from build123d import *

# Parameters (mm, degrees)
SKETCH_1_R      = 2.25
SKETCH_1_R_2    = 4.1
EXTRUDE_1_DEPTH = 1


with BuildPart() as part:
    # 草图1 → 凸台-拉伸1 (new body)
    with BuildSketch(Plane.XY.offset(1)):
        with BuildLine():
            Line((-614.361406616, 5), (-620, 5))
            ThreePointArc((-620, 5), (-622.5, 5.669872981), (-624.330127019, 7.5))
            ThreePointArc((-624.330127019, 7.5), (-625.42820323, 8.598076211), (-626.92820323, 9))
            Line((-626.92820323, 9), (-640, 9))
            ThreePointArc((-640, 9), (-646.363961031, 6.363961031), (-649, 0))
            ThreePointArc((-649, 0), (-600, -49), (-551, 0))
            ThreePointArc((-551, 0), (-553.636038969, 6.363961031), (-560, 9))
            Line((-560, 9), (-573.07179677, 9))
            ThreePointArc((-573.07179677, 9), (-574.57179677, 8.598076211), (-575.669872981, 7.5))
            ThreePointArc((-575.669872981, 7.5), (-577.5, 5.669872981), (-580, 5))
            Line((-580, 5), (-585.638593384, 5))
            ThreePointArc((-585.638593384, 5), (-587.901487472, 3.969596493), (-588.60991889, 1.586206897))
            ThreePointArc((-588.60991889, 1.586206897), (-589.388591149, -4.432606704), (-593.122606779, -9.216911765))
            ThreePointArc((-593.122606779, -9.216911765), (-594.713337054, -9.80559868), (-596.369078113, -9.4375))
            ThreePointArc((-596.369078113, -9.4375), (-600, -8.5), (-603.630921887, -9.4375))
            ThreePointArc((-603.630921887, -9.4375), (-605.286662946, -9.80559868), (-606.877393221, -9.216911765))
            ThreePointArc((-606.877393221, -9.216911765), (-610.611408851, -4.432606704), (-611.39008111, 1.586206897))
            ThreePointArc((-611.39008111, 1.586206897), (-612.098512528, 3.969596493), (-614.361406616, 5))
        make_face()
        with Locations((-640, 0)):
            Circle(SKETCH_1_R, mode=Mode.SUBTRACT)
        with Locations((-600, -30)):
            Circle(SKETCH_1_R_2, mode=Mode.SUBTRACT)
        with Locations((-567.639320225, -23.511410092)):
            Circle(SKETCH_1_R, mode=Mode.SUBTRACT)
        with Locations((-587.639320225, -38.042260652)):
            Circle(SKETCH_1_R, mode=Mode.SUBTRACT)
        with Locations((-612.360679775, -38.042260652)):
            Circle(SKETCH_1_R, mode=Mode.SUBTRACT)
        with Locations((-632.360679775, -23.511410092)):
            Circle(SKETCH_1_R, mode=Mode.SUBTRACT)
        with Locations((-560, 0)):
            Circle(SKETCH_1_R, mode=Mode.SUBTRACT)
    extrude(amount=-EXTRUDE_1_DEPTH)


solid = part.part
Here's how the part is built. I have some questions about the finished solid (model axes, mm). A direction names the side the tool comes from. Round coordinates to 2 decimals unless told otherwise and drop trailing zeros. Order: outer loops, then holes, each group sorted by start corner. A loop starts at its lowest first (then second) coordinate and runs counter-clockwise, first axis right, second up. Notation, with made-up numbers: M -26.5,47 L -11.5,47 A22 ccw -11.5,73 Z; hole C 40,-14.75 d10. An arc over 180 degrees is marked long. One line per question, with ' | ' between items.
1) I'm going to push flat-ended pins straight in: pin 1 Ø2.5 at (x, y) = (-632.36, -23.51) entering from +Z; pin 2 Ø0.5 at (x, z) = (-582.5, 0.5) entering from +Y. Where does each tip first touch, or does it pass through?
Checked values:
pin 1: passes through | pin 2: stops at y = 5
2) On a 3-axis mill with a long thin cutter (end or side, diameter ignored), from which of +Z, -Z, +X, -X, +Y, -Y can I reach the whole of each face in a straight line? I mean faces 4 (the cylindrical face through (-589.356, -4.353, 0.507)), 5 (the cylindrical face through (-577.468, 5.688, 0.507)), 6 (the cylindrical face through (-646.294, 6.434, 0.507)). Say none if no direction works.
Checked values:
face 4: +Z, -Z | face 5: +Z, -Z, +Y | face 6: +Z, -Z, -X, +Y
3) Imagine slicing it at C-C, the plane y = -30. Write out the boundary of the cut face in (x, z).
Checked values:
outline: M -638.74,0 L -604.1,0 L -604.1,1 L -638.74,1 Z; M -595.9,0 L -561.26,0 L -561.26,1 L -595.9,1 Z
4) Imagine slicing it at B-B, the plane z = 0.45. Write out the boundary of the cut face in (x, y).
Checked values:
outline: M -649,0 A49 ccw -551,0 A9 ccw -560,9 L -573.07,9 A3 ccw -575.67,7.5 A5 cw -580,5 L -585.64,5 A3 ccw -588.61,1.59 A11.5 cw -593.12,-9.22 A3 cw -596.37,-9.44 A7.5 ccw -603.63,-9.44 A3 cw -606.88,-9.22 A11.5 cw -611.39,1.59 A3 ccw -614.36,5 L -620,5 A5 cw -624.33,7.5 A3 ccw -626.93,9 L -640,9 A9 ccw Z; hole C -640,0 d4.5; hole C -632.36,-23.51 d4.5; hole C -612.36,-38.04 d4.5; hole C -600,-30 d8.2; hole C -587.64,-38.04 d4.5; hole C -567.64,-23.51 d4.5; hole C -560,0 d4.5
5) I need wall thicknesses on line 1 (Y direction, x = -600, z = 0.95); line 2 (X direction, y = -37, z = 0.35); line 3 (X direction, y = -32.5, z = 0.45). Which ranges of each line are inside material? Lowest first, please.
Checked values:
line 1: y = -49 to -34.1, -25.9 to -8.5 | line 2: x = -632.12 to -614.35, -610.37 to -589.63, -585.65 to -567.88 | line 3: x = -636.67 to -603.25, -596.75 to -563.33
6) Imagine slicing it at D-D, the plane x = -623. Write out the boundary of the cut face in (y, z).
Checked values:
outline: M -43.27,0 L 6,0 L 6,1 L -43.27,1 Z
7) We'd pull the mould along Y, two halves only. Please class faces 1 (the cylindrical face through (-553.566, 6.294, 0.507)), 2 (the cylindrical face through (-614.61, -37.94, 0.51)), 3 (the cylindrical face through (-601.08, -48.99, 0.51)): released by +Y, released by -Y, zero draft, split by the parting line, or undercut.
Checked values:
face 1: released by +Y | face 2: undercut | face 3: released by -Y
8) Imagine slicing it at A-A, the plane x = -600. Write out the boundary of the cut face in (y, z).
Checked values:
outline: M -49,0 L -34.1,0 L -34.1,1 L -49,1 Z; M -25.9,0 L -8.5,0 L -8.5,1 L -25.9,1 Z
